Autodesk Inventor part; units mm, degrees
ref_plane "YZ Plane" through (0, 0, 0) normal (1, 0, 0) x (0, 1, 0)
ref_plane "XZ Plane" through (0, 0, 0) normal (0, 1, 0) x (-1, 0, 0)
ref_plane "XY Plane" through (0, 0, 0) normal (0, 0, 1) x (1, 0, 0)
sketch "Sketch1" plane through (0, 0, 0) normal (0, 1, 0) x (-1, 0, 0)
  line L0 (0, 0) -> (15, 0)
  line L1 (15, 0) -> (15, -120)
  line L2 (0, -120) -> (0, 0)
  arc A0 (0, -120) -> (37.5, -141.6506) centre (25, -120) ccw
  arc A1 (15, -120) -> (30, -128.6603) centre (25, -120) ccw
  line L3 (30, -128.6603) -> (37.5, -141.6506)
  line L4 (25, -120) -> (75, -120) construction
  circle A2 centre (7.5, -45) radius 3
  dimension "d1" = 120
  dimension "d9" = 20
  dimension "d11" = 60
  dimension "d12" = 15
  dimension "d13" = 6
  dimension "d14" = 45
  dimension "d15" = 7.5
extrude "Extrusion1" add sketch "Sketch1" along normal blind 15
properties part number "atividade_14A_garra"
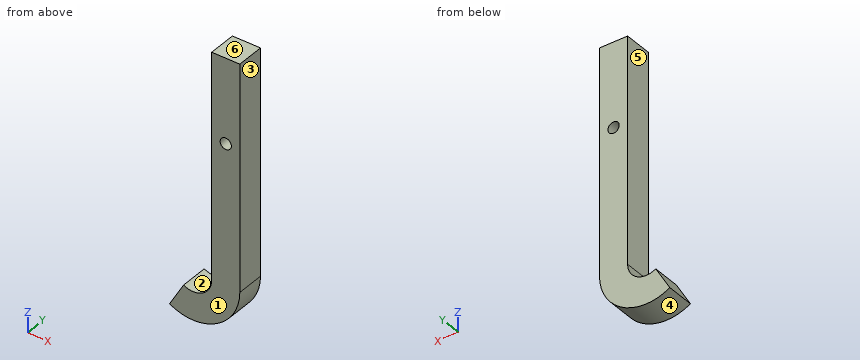
Part model, mm, in its own coordinate system. Face numbers are marked on the shaded views. A direction names the side the tool comes from. Give positions to 0.01 mm unless a question says otherwise; leave off trailing zeros. Loops run counter-clockwise (first coordinate to the right, second up) from the corner with the lowest first, then second, coordinate; pieces in that order, holes last. Notation, with made-up numbers: M 59.5,-24.75 L 113.5,-24.75 A13 cw 113.5,-10.75 Z; hole C 33.25,-3 d6. An arc over 180 degrees is marked long. Return JSON: item names as keys, results as strings.
1) Pull direction X, two halves, no side cores. Call the marked faces 1, 2, 3 and 4: released by +X, released by -X, zero draft, split by the parting line, or undercut.
Calculated:
{"face 1": "zero draft", "face 2": "undercut", "face 3": "released by +X", "face 4": "split by the parting line"}
2) Saw through at C-C, the plane x = -7.5. List the corners of the cut face in (y, z).
Calculated:
{"outline": "M 0,-137.85 L 15,-137.85 L 15,-48 L 0,-48 Z; M 0,-42 L 15,-42 L 15,0 L 0,0 Z"}
3) Flat gauge pins, fed straight in: pin 1 Ø2 at (x, y) = (-28.5, 12) entering from +Z; pin 2 Ø2 at (x, y) = (-20.5, 7.5) entering from -Z. Where does each tip first touch, or does it go through?
Calculated:
{"pin 1": "stops at z = -128.93", "pin 2": "stops at z = -144.75"}
4) 3-axis set-ups, long thin cutter, end or side, ignore diameter. For the marked faces 5 and 6: which of +Z, -Z, +X, -X, +Y, -Y reach the whole face in a straight line?
Calculated:
{"face 5": "+Z, -X, +Y, -Y", "face 6": "+Z, +X, -X, +Y, -Y"}
5) Saw through at A-A, the plane y = 1.5. List the corners of the cut face in (x, z), then the cut area to 3 significant figures.
Calculated:
{"outline": "M -37.5,-141.65 A25 ccw 0,-120 L 0,0 L -15,0 L -15,-120 A10 cw -30,-128.66 Z; hole C -7.5,-45 d6", "area": "2,320 mm2"}
6) Drill centre lines: line 1 (X direction, y = 5.5, z = -12); line 2 (Z direction, x = -7.5, y = 6.25); line 3 (Z direction, x = -6.5, y = 14.25). Where is each one in solid material? Low to high.
Calculated:
{"line 1": "x = -15 to 0", "line 2": "z = -137.85 to -48, -42 to 0", "line 3": "z = -136.82 to -47.83, -42.17 to 0"}
7) Saw through at D-D, the plane x = -21.5. List the corners of the cut face in (y, z), then the cut area to 3 significant figures.
Calculated:
{"outline": "M 0,-144.75 L 15,-144.75 L 15,-129.37 L 0,-129.37 Z", "area": "231 mm2"}
8) Saw through at B-B, the plane z = -45. List the corners of the cut face in (x, y).
Calculated:
{"outline": "M -15,0 L -10.5,0 L -10.5,15 L -15,15 Z; M -4.5,0 L 0,0 L 0,15 L -4.5,15 Z"}
